Verification items for the finished model (mm, model axes). A direction names the side the tool comes from. Coordinates: 2 decimals unless noted, no trailing zeros. Write each loop counter-clockwise with the first axis right and the second up, starting at its lowest first coordinate (ties: lowest second). Pieces come first, ordered by that corner, then holes. Notation, with made-up numbers: (9.25, 23) -> (15.25, 23) arc R19 ccw to (15.25, 27) -> close; hole circle Ø11 at (-8, 69.25). An arc over 180 degrees is marked (long way). Answer in a Markdown table with one row per item.
Autodesk Inventor part; units mm, degrees
ref_plane "YZ Plane" through (0, 0, 0) normal (1, 0, 0) x (0, 1, 0)
ref_plane "XZ Plane" through (0, 0, 0) normal (0, 1, 0) x (-1, 0, 0)
ref_plane "XY Plane" through (0, 0, 0) normal (0, 0, 1) x (1, 0, 0)
sketch "Sketch1" plane through (0, 0, 0) normal (0, 1, 0) x (-1, 0, 0)
  line L0 (-39.6875, 39.6875) -> (39.6875, 39.6875)
  line L1 (39.6875, 39.6875) -> (39.6875, -39.6875)
  line L2 (39.6875, -39.6875) -> (-39.6875, -39.6875)
  line L3 (-39.6875, -39.6875) -> (-39.6875, 39.6875)
  line L4 (-39.6875, 39.6875) -> (39.6875, -39.6875) construction
  line L5 (39.6875, 39.6875) -> (-39.6875, -39.6875) construction
  line L6 (-35.8775, 35.8775) -> (35.8775, 35.8775)
  line L7 (35.8775, 35.8775) -> (35.8775, -35.8775)
  line L8 (35.8775, -35.8775) -> (-35.8775, -35.8775)
  line L9 (-35.8775, -35.8775) -> (-35.8775, 35.8775)
  line L10 (-35.8775, 35.8775) -> (35.8775, -35.8775) construction
  line L11 (35.8775, 35.8775) -> (-35.8775, -35.8775) construction
  line L12 (0, -55.5625) -> (0, 55.5625)
  point P0 (0, 0)
  dimension "d0" = 3.81
  dimension "d10" = 79.375
  dimension "d11" = 45
extrude "Extrusion1" add sketch "Sketch1" along normal blind 80.772 contours L0 L12 L6 L9 L8 L2 L3 | L0 L1 L2 L12 L8 L7 L6
extrude "Extrusion2" add sketch "Sketch1" along normal blind 9.652 contours L12 L8 L9 L6 | L6 L7 L8 L12
fillet "Fillet1" radius 3.81 12 edges at (-39.6875, 40.386, 39.6875) (-35.8775, 45.212, 35.8775) (-39.6875, 40.386, -39.6875) (-35.8775, 45.212, -35.8775) (35.8775, 45.212, -35.8775) (39.6875, 40.386, -39.6875) (35.8775, 45.212, 35.8775) (39.6875, 40.386, 39.6875) (-35.8775, 9.652, 0) (0, 9.652, 35.8775) (0, 9.652, -35.8775) (35.8775, 9.652, 0)
properties part number "CandleHolder-3" material "Glass"
1. Depth check by flat-ended pin: P1, Ø6, axis at x = -13, z = -12.5, coming from the -Y side. Enter the tip coordinate at first touch or a pass-through.
Geometry says:
| item | result |
|---|---|
| P1 | y = 0 |
2. Section check C-C, the plane z = 27. Record the boundary of the cut face in (x, y), plus the area to 3 significant figures.
Geometry says:
| item | result |
|---|---|
| outline | (-39.69, 0) -> (39.69, 0) -> (39.69, 80.77) -> (35.88, 80.77) -> (35.88, 13.46) arc R3.81 cw to (32.07, 9.65) -> (-32.07, 9.65) arc R3.81 cw to (-35.88, 13.46) -> (-35.88, 80.77) -> (-39.69, 80.77) -> close |
| area | 1,310 mm^2 |
3. Section check A-A, the plane x = 16. Record the boundary of the cut face in (y, z).
Geometry says:
| item | result |
|---|---|
| outline | (0, -39.69) -> (80.77, -39.69) -> (80.77, -35.88) -> (13.46, -35.88) arc R3.81 cw to (9.65, -32.07) -> (9.65, 32.07) arc R3.81 cw to (13.46, 35.88) -> (80.77, 35.88) -> (80.77, 39.69) -> (0, 39.69) -> close |
4. Mould release check, pull along X, two halves, no side actions. Record for faces 1 (the flat face through (-39.688, 40, 1)), 2 (the flat face through (-35.878, 47, 0)), 3 (the flat face through (0, 80.772, 38)), 4 (the flat face through (0, 47, -35.878)): released by +X, released by -X, zero draft, split by the parting line, or undercut.
Geometry says:
| item | result |
|---|---|
| face 1 | released by -X |
| face 2 | undercut |
| face 3 | zero draft |
| face 4 | undercut |
5. Tool access check on faces 5 (the cylindrical face through (38.54, 40.95, 38.6)), 6 (the cylindrical face through (34.79, 47.59, -34.73)). Record the directions out of +Z, -Z, +X, -X, +Y, -Y that give a thin tool (end or side, any length) a straight path to the whole face; none if there is none.
Geometry says:
| item | result |
|---|---|
| face 5 | +Z, +X, +Y, -Y |
| face 6 | +Y |
6. Thickness scan on line 1 (Z direction, x = -21, y = 29.5); line 2 (X direction, y = 13, z = 23.5). Record the ranges inside material, lowest first. Write a range as from..to.
Geometry says:
| item | result |
|---|---|
| line 1 | -39.69..-35.88, 35.88..39.69 |
| line 2 | -39.69..-35.85, 35.85..39.69 |
7. Section check B-B, the plane y = 40. Record the boundary of the cut face in (x, z), plus the area to 3 significant figures.
Geometry says:
| item | result |
|---|---|
| outline | (-39.69, -35.88) arc R3.81 ccw to (-35.88, -39.69) -> (35.88, -39.69) arc R3.81 ccw to (39.69, -35.88) -> (39.69, 35.88) arc R3.81 ccw to (35.88, 39.69) -> (-35.88, 39.69) arc R3.81 ccw to (-39.69, 35.88) -> close; hole (-35.88, -32.07) arc R3.81 ccw to (-32.07, -35.88) -> (32.07, -35.88) arc R3.81 ccw to (35.88, -32.07) -> (35.88, 32.07) arc R3.81 ccw to (32.07, 35.88) -> (-32.07, 35.88) arc R3.81 ccw to (-35.88, 32.07) -> close |
| area | 1,150 mm^2 |
